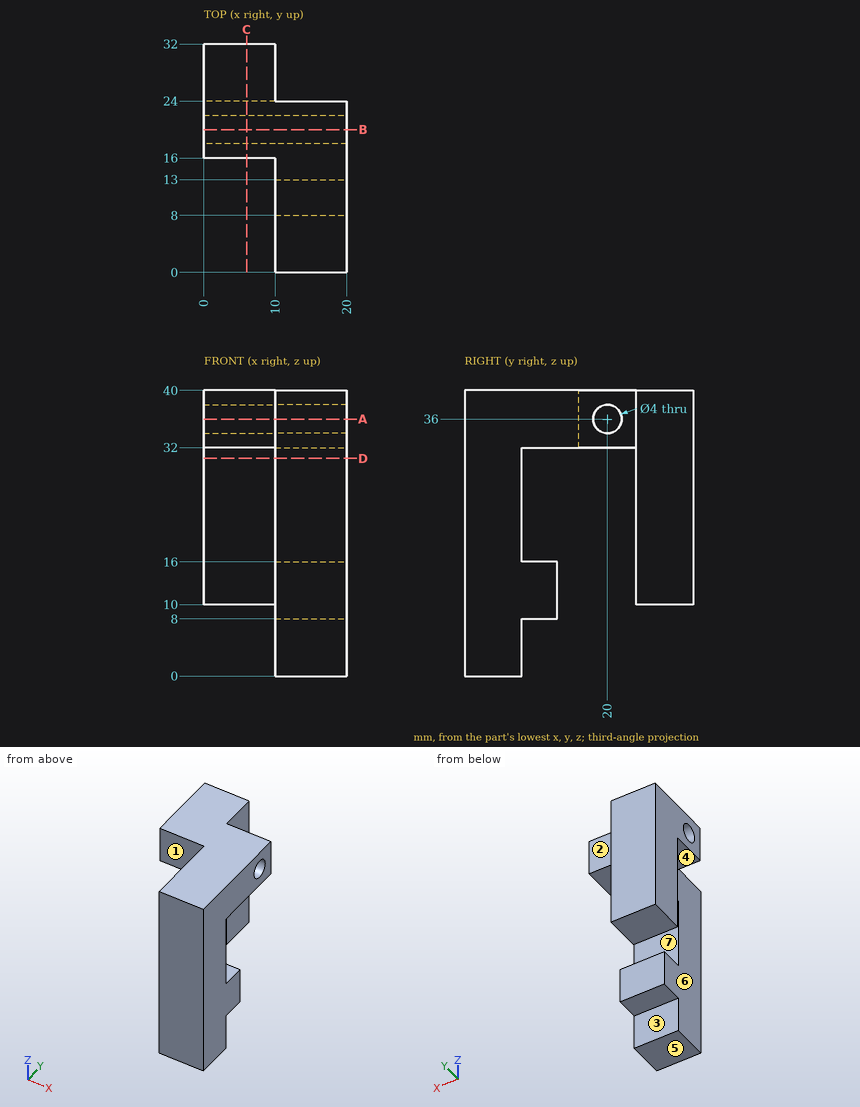
Check sheet for the drawn part. Datum: minimum x, y, z corner. Units: mm. A direction names the side the tool comes from. Give positions to 0.01 mm unless a question says otherwise; leave off trailing zeros. Write each loop counter-clockwise with the first axis right and the second up, starting at its lowest first coordinate (ties: lowest second). Pieces come first, ordered by that corner, then holes.
(1) Material ranges on line 1 (Y direction, x = 14, z = 36); line 2 (Z direction, x = 6.5, y = 20); line 3 (Y direction, x = 6.75, z = 36), recorded low to high.
(2) Cross-section at D-D (z = 30.5). Enter the section's corners in (x, y), plus the area to 3 significant figures.
(3) Cross-section at A-A (z = 36). Enter the section's corners in (x, y), plus the area to 3 significant figures.
(4) Access from +Z, -Z, +X, -X, +Y, -Y to the whole of each face (thin tool, end or side, straight path). Record for the marked faces 1, 2, 3 and 4.
(5) Cross-section at B-B (y = 20). Enter the section's corners in (x, z).
(6) Gauge pin test, flat ends, axial feed: pin 1 (3 mm diameter, centred on x = 15.5, z = 13, fed in from +Y); pin 2 (5 mm diameter, centred on y = 5, z = 20, fed in from -X); pin 3 (2.5 mm diameter, centred on x = 14, z = 36.5, fed in from +Y); pin 4 (3.5 mm diameter, centred on y = 20, z = 36, fed in from -X). Record the tip position at first contact, or that the pin passes through.
(7) Cross-section at C-C (x = 6). Enter the section's corners in (y, z), plus the area to 3 significant figures.
(8) Mould release check, pull along Z, two halves, no side actions. Record for the marked faces 5, 6 and 7: +Z half, -Z half, draft (parallel to the pull), parting line (faces both ways), or undercut.
Worked out:
1. line 1: y = 0 to 18, 22 to 24
1. line 2: z = 32 to 34, 38 to 40
1. line 3: y = 16 to 18, 22 to 32
2. outline: (0, 24) - (10, 24) - (10, 32) - (0, 32) - close; (10, 0) - (20, 0) - (20, 8) - (10, 8) - close
2. area: 160 mm2
3. outline: (0, 16) - (10, 16) - (10, 0) - (20, 0) - (20, 18) - (0, 18) - close; (0, 22) - (20, 22) - (20, 24) - (10, 24) - (10, 32) - (0, 32) - close
3. area: 320 mm2
4. face 1: +Z, -Z, -X, -Y
4. face 2: +Z, -Z, +X, +Y
4. face 3: -Z, +X, -X, +Y
4. face 4: +X, -X
5. outline: (0, 32) - (20, 32) - (20, 34) - (0, 34) - close; (0, 38) - (20, 38) - (20, 40) - (0, 40) - close
6. pin 1: stops at y = 13
6. pin 2: stops at x = 10
6. pin 3: stops at y = 24
6. pin 4: passes through
7. outline: (16, 32) - (24, 32) - (24, 10) - (32, 10) - (32, 40) - (16, 40) - close; hole circle Ø4 at (20, 36)
7. area: 291 mm2
8. face 5: -Z half
8. face 6: draft
8. face 7: undercut
